from build123d import *

# Parameters (mm, degrees)
SKETCH1_W           = 60
SKETCH1_H           = 30
SKETCH1_W_2         = 41.5
SKETCH1_H_2         = 21.5
BOSS_EXTRUDE1_DEPTH = 27
SKETCH2_R           = 50
BOSS_EXTRUDE2_DEPTH = 5
FILLET2_R           = 10
SKETCH6_R           = 1
CUT_EXTRUDE2_DEPTH  = 15
SKETCH7_W           = 41.5
SKETCH7_H           = 21.5
CUT_EXTRUDE3_DEPTH  = 69
SKETCH8_W           = 10
SKETCH8_H           = 6
CUT_EXTRUDE4_DEPTH  = 75
SKETCH10_W          = 74.59493419
SKETCH10_H          = 6
CUT_EXTRUDE5_DEPTH  = 3
SKETCH11_R          = 2
CUT_EXTRUDE6_DEPTH  = 16
BOSS_EXTRUDE3_DEPTH = 5
SKETCH13_R          = 2.5
SKETCH13_R_2        = 1
BOSS_EXTRUDE4_DEPTH = 4
SKETCH14_R          = 2.5
SKETCH14_R_2        = 1
BOSS_EXTRUDE5_DEPTH = 4
SKETCH15_R          = 2.5
SKETCH15_R_2        = 1
BOSS_EXTRUDE6_DEPTH = 4
BOSS_EXTRUDE8_DEPTH = 17.5
SKETCH17_W          = 3
SKETCH17_H          = 6
CUT_EXTRUDE7_DEPTH  = 17.5
SKETCH18_W          = 1.640081146
SKETCH18_H          = 6
CUT_EXTRUDE8_DEPTH  = 3
SKETCH20_W          = 13
SKETCH20_H          = 15.827650688
CUT_EXTRUDE9_DEPTH  = 25
SKETCH21_W          = 10
SKETCH21_H          = 3
CUT_EXTRUDE10_DEPTH = 13.5
SKETCH23_W          = 13
SKETCH23_H          = 3
SKETCH23_W_2        = 10
BOSS_EXTRUDE9_DEPTH = 1.75
FILLET3_R           = 1
SKETCH24_R          = 2
CUT_EXTRUDE11_DEPTH = 17
SKETCH25_W          = 10.72256849
SKETCH25_H          = 6
CUT_EXTRUDE12_DEPTH = 3
FILLET4_R           = 2


with BuildPart() as part:
    # Sketch1 → Boss-Extrude1 (new body)
    with BuildSketch(Plane.XY):
        Rectangle(SKETCH1_W, SKETCH1_H)
        Rectangle(SKETCH1_W_2, SKETCH1_H_2, mode=Mode.SUBTRACT)
    extrude(amount=BOSS_EXTRUDE1_DEPTH)

    # Sketch2 → Boss-Extrude2 (add)
    with BuildSketch(Plane.XY.offset(27)):
        Circle(SKETCH2_R)
    extrude(amount=BOSS_EXTRUDE2_DEPTH)

    # Fillet2
    fillet2_edges = [part.edges().sort_by_distance(p)[0] for p in [
        (30, 0, 27),
        (0, 15, 27),
        (-30, 0, 27),
        (0, -15, 27),
    ]]
    fillet(fillet2_edges, radius=FILLET2_R)

    # Sketch6 → Cut-Extrude2 (cut)
    with BuildSketch(Plane(origin=(0, 0, 0), x_dir=(-1, 0, 0), z_dir=(0, 0, -1))):
        with Locations((24.4, 5)):
            Circle(SKETCH6_R)
        with Locations((-24.4, 5)):
            Circle(SKETCH6_R)
        with Locations((24.4, -5)):
            Circle(SKETCH6_R)
        with Locations((-24.4, -5)):
            Circle(SKETCH6_R)
    extrude(amount=-CUT_EXTRUDE2_DEPTH, mode=Mode.SUBTRACT)

    # Sketch7 → Cut-Extrude3 (cut)
    with BuildSketch(Plane(origin=(0, 0, 0), x_dir=(-1, 0, 0), z_dir=(0, 0, -1))):
        Rectangle(SKETCH7_W, SKETCH7_H)
    extrude(amount=-CUT_EXTRUDE3_DEPTH, mode=Mode.SUBTRACT)

    # Sketch8 → Cut-Extrude4 (cut)
    with BuildSketch(Plane(origin=(0, 0, 0), x_dir=(-1, 0, 0), z_dir=(0, 0, -1))):
        with Locations((20.75, 0)):
            Rectangle(SKETCH8_W, SKETCH8_H)
    extrude(amount=-CUT_EXTRUDE4_DEPTH, mode=Mode.SUBTRACT)

    # Sketch10 → Cut-Extrude5 (cut)
    with BuildSketch(Plane.XY.offset(32)):
        with Locations((37.297467095, 0)):
            Rectangle(SKETCH10_W, SKETCH10_H)
    extrude(amount=-CUT_EXTRUDE5_DEPTH, mode=Mode.SUBTRACT)

    # Sketch11 → Cut-Extrude6 (cut)
    with BuildSketch(Plane(origin=(0, 0, 27), x_dir=(-1, 0, 0), z_dir=(0, 0, -1))):
        with Locations((45, 0)):
            Circle(SKETCH11_R)
        with Locations((-22.5, 38.97114317)):
            Circle(SKETCH11_R)
        with Locations((-22.5, -38.97114317)):
            Circle(SKETCH11_R)
    extrude(amount=-CUT_EXTRUDE6_DEPTH, mode=Mode.SUBTRACT)

    # Sketch12 → Boss-Extrude3 (add)
    with BuildSketch(Plane(origin=(0, 0, 27), x_dir=(-1, 0, 0), z_dir=(0, 0, -1))):
        with BuildLine():
            Line((0, -50), (-125, -50))
            Line((-125, -50), (-125, 50))
            Line((-125, 50), (0, 50))
            ThreePointArc((0, 50), (-50, 0), (0, -50))
        make_face()
    extrude(amount=-BOSS_EXTRUDE3_DEPTH)

    # Sketch13 → Boss-Extrude4 (add)
    with BuildSketch(Plane(origin=(0, 0, 27), x_dir=(-1, 0, 0), z_dir=(0, 0, -1))):
        with Locations((-104.5, -20)):
            Circle(SKETCH13_R)
        with Locations((-104.5, -20)):
            Circle(SKETCH13_R_2, mode=Mode.SUBTRACT)
    extrude(amount=BOSS_EXTRUDE4_DEPTH)

    # Sketch14 → Boss-Extrude5 (add)
    with BuildSketch(Plane(origin=(0, 0, 27), x_dir=(-1, 0, 0), z_dir=(0, 0, -1))):
        with Locations((-56.25, -21.25)):
            Circle(SKETCH14_R)
        with Locations((-56.25, -21.25)):
            Circle(SKETCH14_R_2, mode=Mode.SUBTRACT)
    extrude(amount=BOSS_EXTRUDE5_DEPTH)

    # Sketch15 → Boss-Extrude6 (add)
    with BuildSketch(Plane(origin=(0, 0, 27), x_dir=(-1, 0, 0), z_dir=(0, 0, -1))):
        with Locations((-61.34, 30.85)):
            Circle(SKETCH15_R)
        with Locations((-61.34, 30.85)):
            Circle(SKETCH15_R_2, mode=Mode.SUBTRACT)
        with Locations((-89.2, 30.85)):
            Circle(SKETCH15_R)
        with Locations((-89.2, 30.85)):
            Circle(SKETCH15_R_2, mode=Mode.SUBTRACT)
    extrude(amount=BOSS_EXTRUDE6_DEPTH)

    # Sketch16 → Boss-Extrude8 (add)
    with BuildSketch(Plane(origin=(0, 0, 27), x_dir=(-1, 0, 0), z_dir=(0, 0, -1))):
        Polygon((-112.05, 38.25), (-48.55, 38.25), (-48.55, -38.75), (-112.05, -38.75), (-112.05, 7.205124567), align=None)
        Polygon((-109.05, 7.205124567), (-109.05, 35.25), (-51.55, 35.25), (-51.55, -35.75), (-109.05, -35.75), align=None, mode=Mode.SUBTRACT)
    extrude(amount=BOSS_EXTRUDE8_DEPTH)

    # Sketch17 → Cut-Extrude7 (cut)
    with BuildSketch(Plane(origin=(0, 0, 27), x_dir=(-1, 0, 0), z_dir=(0, 0, -1))):
        with Locations((-53.05, 0)):
            Rectangle(SKETCH17_W, SKETCH17_H)
    extrude(amount=-CUT_EXTRUDE7_DEPTH, mode=Mode.SUBTRACT)

    # Sketch18 → Cut-Extrude8 (cut)
    with BuildSketch(Plane.XY.offset(32)):
        with Locations((50.729959427, 0)):
            Rectangle(SKETCH18_W, SKETCH18_H)
    extrude(amount=-CUT_EXTRUDE8_DEPTH, mode=Mode.SUBTRACT)

    # Sketch20 → Cut-Extrude9 (cut)
    with BuildSketch(Plane(origin=(0, 0, 23), x_dir=(-1, 0, 0), z_dir=(0, 0, -1))):
        with Locations((-91.75, -35.907506038)):
            Rectangle(SKETCH20_W, SKETCH20_H)
    extrude(amount=CUT_EXTRUDE9_DEPTH, mode=Mode.SUBTRACT)

    # Sketch21 → Cut-Extrude10 (cut)
    with BuildSketch(Plane(origin=(0, 0, 9.5), x_dir=(-1, 0, 0), z_dir=(0, 0, -1))):
        with Locations((-61.43, -37.25)):
            Rectangle(SKETCH21_W, SKETCH21_H)
    extrude(amount=-CUT_EXTRUDE10_DEPTH, mode=Mode.SUBTRACT)

    # Sketch23 → Boss-Extrude9 (add)
    with BuildSketch(Plane(origin=(0, 0, 23), x_dir=(-1, 0, 0), z_dir=(0, 0, -1))):
        with Locations((-91.75, -37.25)):
            Rectangle(SKETCH23_W, SKETCH23_H)
        with Locations((-61.43, -37.25)):
            Rectangle(SKETCH23_W_2, SKETCH23_H)
    extrude(amount=BOSS_EXTRUDE9_DEPTH)

    # Fillet3
    fillet3_edges = [part.edges().sort_by_distance(p)[0] for p in [
        (112.05, 38.25, 18.25),
        (112.05, -38.75, 18.25),
        (48.55, -38.75, 18.25),
        (48.55, 38.25, 18.25),
    ]]
    fillet(fillet3_edges, radius=FILLET3_R)

    # Sketch24 → Cut-Extrude11 (cut)
    with BuildSketch(Plane(origin=(0, 0, 27), x_dir=(-1, 0, 0), z_dir=(0, 0, -1))):
        with Locations((-117.5, 38.97114317)):
            Circle(SKETCH24_R)
        with Locations((-117.5, -38.97114317)):
            Circle(SKETCH24_R)
    extrude(amount=-CUT_EXTRUDE11_DEPTH, mode=Mode.SUBTRACT)

    # Sketch25 → Cut-Extrude12 (cut)
    with BuildSketch(Plane(origin=(0, 0, 0), x_dir=(-1, 0, 0), z_dir=(0, 0, -1))):
        with Locations((25.75, 0)):
            Rectangle(SKETCH25_W, SKETCH25_H)
    extrude(amount=-CUT_EXTRUDE12_DEPTH, mode=Mode.SUBTRACT)

    # Fillet4
    fillet4_edges = [part.edges().sort_by_distance(p)[0] for p in [
        (-25.75, 0, 3),
        (51.55, 0, 29),
    ]]
    fillet(fillet4_edges, radius=FILLET4_R)


solid = part.part
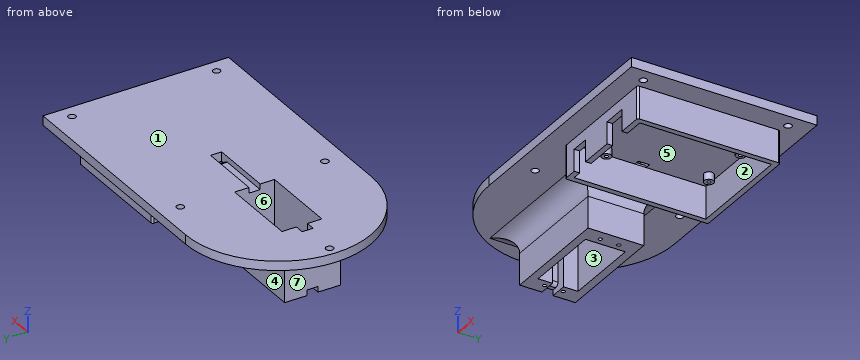
Work out the finished part from the listing and answer in its coordinate system (mm). Face numbers are marked on the shaded views. A direction names the side the tool comes from. Round coordinates to 2 decimals unless told otherwise and drop trailing zeros. Write each loop counter-clockwise with the first axis right and the second up, starting at its lowest first coordinate (ties: lowest second). Pieces come first, ordered by that corner, then holes.
1) The mould has two halves that part along Y. Classify the marked faces 1, 2, 3 and 4: pulls with the +Y half, pulls with the -Y half, needs draft (parallel to the pull), parting line crosses it, or undercut.
2) A cutting plane is placed at A-A (z = 12). Give the number of separate pieces and of enclosed holes in the cut face, plus the area to 3 significant figures.
3) A cutting plane is placed at B-B (y = -13). Give the vertices of the cut face in (x, z), plus the area to 3 significant figures.
4) Straight lines are drawn through the part: line 1 (Y direction, x = -24.4, z = 9.5); line 2 (X direction, y = 10, z = 3); line 3 (X direction, y = 9, z = 24). For each, find the intervals that lie inside material, in ascending order.
5) A tool of negligible diameter and unlimited length cuts with its end or side. For the marked faces 5, 6 and 7, from which of +Z, -Z, +X, -X, +Y, -Y can it reach the whole face along a straight path? Write none if from no direction.
6) A cutting plane is placed at C-C (y = 19.5). Give the vertices of the cut face in (x, z).
7) Given pin 1 Ø1.6 at (x, y) = (104.5, -20) entering from -Z; pin 2 Ø14 at (x, z) = (72.5, 15) entering from -Y; pin 3 Ø1.2 at (x, y) = (-24.4, 5) entering from -Z, each flat-ended and moving along its own axis, determine where each tip first touches the part or whether it passes through.
Completed:
1. face 1: needs draft
1. face 2: undercut
1. face 3: undercut
1. face 4: pulls with the +Y half
2. separate pieces: 3
2. enclosed holes: 5
2. area: 1,600 mm2
3. outline: (-48.28, 27) - (-40, 27) arc R10 cw to (-30, 17) - (-30, 0) - (30, 0) - (30, 17) arc R10 cw to (40, 27) - (48.55, 27) - (48.55, 9.5) - (51.55, 9.5) - (51.55, 27) - (109.05, 27) - (109.05, 9.5) - (112.05, 9.5) - (112.05, 27) - (125, 27) - (125, 32) - (-48.28, 32) - close
3. area: 2,630 mm2
4. line 1: y = -15 to -6, -4 to -3, 3 to 4, 6 to 15
4. line 2: x = -30 to -20.75, 20.75 to 30
4. line 3: x = -32.86 to -20.75, 20.75 to 32.86, 48.55 to 51.55, 109.05 to 112.05
5. face 5: -Z
5. face 6: +Z, -Z
5. face 7: -Z, -X, +Y, -Y
6. outline: (-46.04, 27) - (-40, 27) arc R10 cw to (-34.5, 25.35) - (34.5, 25.35) arc R10 cw to (40, 27) - (48.55, 27) - (48.55, 9.5) - (51.55, 9.5) - (51.55, 27) - (109.05, 27) - (109.05, 9.5) - (112.05, 9.5) - (112.05, 27) - (125, 27) - (125, 32) - (-46.04, 32) - close
7. pin 1: stops at z = 27
7. pin 2: stops at y = -38.75
7. pin 3: stops at z = 15
